from build123d import *

# Parameters (mm, degrees)
SKETCH_1_W          = 55
SKETCH_1_H          = 25
EXTRUDE_1_DEPTH     = 119.5
SKETCH_3_W          = 2
SKETCH_3_H          = 25
EXTRUDE_2_DEPTH     = 10
EXTRUDE_3_DEPTH     = 25
SKETCH_6_R          = 1.6
CUT_EXTRUDE_2_DEPTH = 131.118748168
SKETCH_7_W          = 2
SKETCH_7_H          = 25
EXTRUDE_4_DEPTH     = 10
EXTRUDE_5_DEPTH     = 25
SKETCH_9_R          = 1.6
CUT_EXTRUDE_3_DEPTH = 131.118748168
SKETCH_10_W         = 55
SKETCH_10_H         = 4
CUT_EXTRUDE_4_DEPTH = 20
SKETCH_12_W         = 41
SKETCH_12_H         = 21
CUT_EXTRUDE_5_DEPTH = 20
SKETCH_13_R         = 1.4
CUT_EXTRUDE_6_DEPTH = 10
SKETCH_15_R         = 1.4
CUT_EXTRUDE_7_DEPTH = 10


with BuildPart() as part:
    # ｽｹｯﾁ1 → ﾎﾞｽ - 押し出し1 (new body)
    with BuildSketch(Plane.XY):
        with Locations((14.77105538, -7.308467742)):
            Rectangle(SKETCH_1_W, SKETCH_1_H)
    extrude(amount=EXTRUDE_1_DEPTH)

    # ｽｹｯﾁ3 → ﾎﾞｽ - 押し出し2 (add)
    with BuildSketch(Plane(origin=(42.27105538, 0, 0), x_dir=(0, 0, -1), z_dir=(1, 0, 0))):
        with Locations((-1, -7.308467742)):
            Rectangle(SKETCH_3_W, SKETCH_3_H)
    extrude(amount=EXTRUDE_2_DEPTH)

    # ｽｹｯﾁ5 → ﾎﾞｽ - 押し出し3 (add, through all)
    with BuildSketch(Plane(origin=(0, 5.191532258, 0), x_dir=(1, 0, 0), z_dir=(0, 1, 0))):
        Polygon((42.27105538, -5), (45.27105538, -2), (42.27105538, -2), align=None)
    extrude(amount=-EXTRUDE_3_DEPTH)

    # ｽｹｯﾁ6 → ｶｯﾄ - 押し出し2 (cut, through all)
    with BuildSketch(Plane.XY.offset(2)):
        with Locations((48.77105538, 1.691532258)):
            Circle(SKETCH_6_R)
        with Locations((48.77105538, -16.308467742)):
            Circle(SKETCH_6_R)
    extrude(amount=-CUT_EXTRUDE_2_DEPTH, mode=Mode.SUBTRACT)

    # ｽｹｯﾁ7 → ﾎﾞｽ - 押し出し4 (add)
    with BuildSketch(Plane.ZY.offset(12.72894462)):
        with Locations((1, -7.308467742)):
            Rectangle(SKETCH_7_W, SKETCH_7_H)
    extrude(amount=EXTRUDE_4_DEPTH)

    # ｽｹｯﾁ8 → ﾎﾞｽ - 押し出し5 (add, through all)
    with BuildSketch(Plane.XZ.offset(19.808467742)):
        Polygon((-12.72894462, 5), (-15.72894462, 2), (-12.72894462, 2), align=None)
    extrude(amount=-EXTRUDE_5_DEPTH)

    # ｽｹｯﾁ9 → ｶｯﾄ - 押し出し3 (cut, through all)
    with BuildSketch(Plane.XY.offset(2)):
        with Locations((-19.22894462, -16.308467742)):
            Circle(SKETCH_9_R)
        with Locations((-19.22894462, 1.691532258)):
            Circle(SKETCH_9_R)
    extrude(amount=-CUT_EXTRUDE_3_DEPTH, mode=Mode.SUBTRACT)

    # ｽｹｯﾁ10 → ｶｯﾄ - 押し出し4 (cut)
    with BuildSketch(Plane.XY.offset(119.5)):
        with Locations((14.77105538, -17.808467742)):
            Rectangle(SKETCH_10_W, SKETCH_10_H)
    extrude(amount=-CUT_EXTRUDE_4_DEPTH, mode=Mode.SUBTRACT)

    # ｽｹｯﾁ12 → ｶｯﾄ - 押し出し5 (cut)
    with BuildSketch(Plane.XY.offset(119.5)):
        with Locations((14.77105538, -5.308467742)):
            Rectangle(SKETCH_12_W, SKETCH_12_H)
    extrude(amount=-CUT_EXTRUDE_5_DEPTH, mode=Mode.SUBTRACT)

    # ｽｹｯﾁ13 → ｶｯﾄ - 押し出し6 (cut)
    with BuildSketch(Plane.XZ.offset(15.808467742)):
        with Locations((39.27105538, 104.5)):
            Circle(SKETCH_13_R)
        with Locations((39.27105538, 114.5)):
            Circle(SKETCH_13_R)
    extrude(amount=-CUT_EXTRUDE_6_DEPTH, mode=Mode.SUBTRACT)

    # ｽｹｯﾁ15 → ｶｯﾄ - 押し出し7 (cut)
    with BuildSketch(Plane(origin=(0, -15.808467742, 0), x_dir=(-1, 0, 0), z_dir=(0, -1, 0))):
        with Locations(Location((9.72894462, -104.5, 0), (0, 0, 180))):
            Circle(SKETCH_15_R)
        with Locations(Location((9.72894462, -114.5, 0), (0, 0, 180))):
            Circle(SKETCH_15_R)
    extrude(amount=-CUT_EXTRUDE_7_DEPTH, mode=Mode.SUBTRACT)


solid = part.part
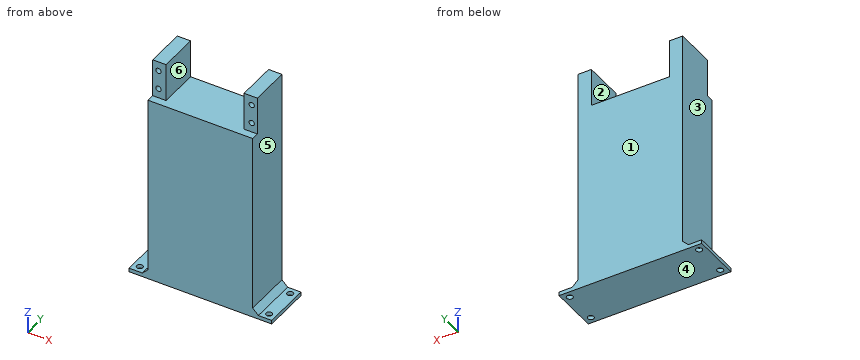
Source: CAD feature listing. Evaluate the final solid. Frame: model axes, mm. Face numbers are marked on the shaded views. A direction names the side the tool comes from. Give positions to 0.01 mm unless a question says otherwise; leave off trailing zeros. Write each loop counter-clockwise with the first axis right and the second up, starting at its lowest first coordinate (ties: lowest second). Pieces come first, ordered by that corner, then holes. Notation, with made-up numbers: (42.5, -22) - (100.5, -22) arc R12 cw to (100.5, 1) - close; hole circle Ø7 at (14, 80). An arc over 180 degrees is marked (long way). Write item = value, one per line. Start each with the question number.
Q1. Cut plane B-B, the plane z = 13. Return loops of the section in (x, y).
Q2. Cut plane C-C, the plane x = 29.5. Return loops of the section in (y, z), then the cut area to 3 significant figures.
Q3. Cut plane A-A, the plane z = 114.5. Return loops of the section in (x, y), then the cut area to 3 significant figures.
Q4. Reachability of the marked faces 1 and 2 from +Z, -Z, +X, -X, +Y, -Y: full face, straight path, thin tool, end or side. Return the list, or none.
Q5. Draft query along X for the marked faces 3, 4, 5 and 6. Return one class per face: +X half, -X half, draft (parallel to the pull), parting line (faces both ways), or undercut.
Q6. Material intervals for probe 1 along X at (y, z) = (-9.5, 110); probe 2 along X at (y, z) = (-6, 113.5); probe 3 along X at (y, z) = (-12, 13.5), sorted ascending.
Q7. Pin query (flat end, axial travel): pin 1 Ø7.5 at (x, y) = (47.5, -10.5) entering from +Z; pin 2 Ø6 at (y, z) = (-12, 48) entering from +X; pin 3 Ø3 at (x, z) = (39.27, 114.5) entering from -Y. Return the tip coordinate at first contact, or that it passes through.
Computed values:
q1.outline = (-12.73, -19.81) - (42.27, -19.81) - (42.27, 5.19) - (-12.73, 5.19) - close
q2.outline = (-19.81, 0) - (5.19, 0) - (5.19, 99.5) - (-19.81, 99.5) - close
q2.area = 2,490 mm²
q3.outline = (-12.73, -15.81) - (-11.13, -15.81) - (-11.13, -5.81) - (-8.33, -5.81) - (-8.33, -15.81) - (-5.73, -15.81) - (-5.73, 5.19) - (-12.73, 5.19) - close; (35.27, -15.81) - (37.87, -15.81) - (37.87, -5.81) - (40.67, -5.81) - (40.67, -15.81) - (42.27, -15.81) - (42.27, 5.19) - (35.27, 5.19) - close
q3.area = 238 mm²
q4.face_1 = +Z, -Z, +X, -X, +Y
q4.face_2 = +Z, +Y, -Y
q5.face_3 = -X half
q5.face_4 = draft
q5.face_5 = +X half
q5.face_6 = undercut
q6.probe_1 = -12.73 to -5.73, 35.27 to 42.27
q6.probe_2 = -12.73 to -10.71, -8.75 to -5.73, 35.27 to 38.29, 40.25 to 42.27
q6.probe_3 = -12.73 to 42.27
q7.pin_1 = 3.52
q7.pin_2 = 42.27
q7.pin_3 = -15.81
